Check sheet for the drawn part. Datum: minimum x, y, z corner. Units: mm. Coordinates: 2 decimals unless noted, no trailing zeros. Write each loop counter-clockwise with the first axis right and the second up, starting at its lowest first coordinate (ties: lowest second). Pieces come first, ordered by that corner, then holes. Notation, with made-up numbers: (83, 47) -> (93, 47) arc R20 cw to (93, 71) -> close; hole circle Ø3 at (25.25, 35.5). An arc over 180 degrees is marked (long way). Answer in a Markdown table with one row per item. Add a question column.
1. Scan lines: L1, parallel to X at y = 7, z = 1.75; L2, parallel to Y at x = 8.5, z = 0.6. Record each from-to range of solid material in increasing order. Write a range as from..to.
2. Cross-section at B-B on y = 1. Record the cut outline in (x, z).
3. Cross-section at A-A on y = 5. Record the cut outline in (x, z), and give its area (3 significant figures).
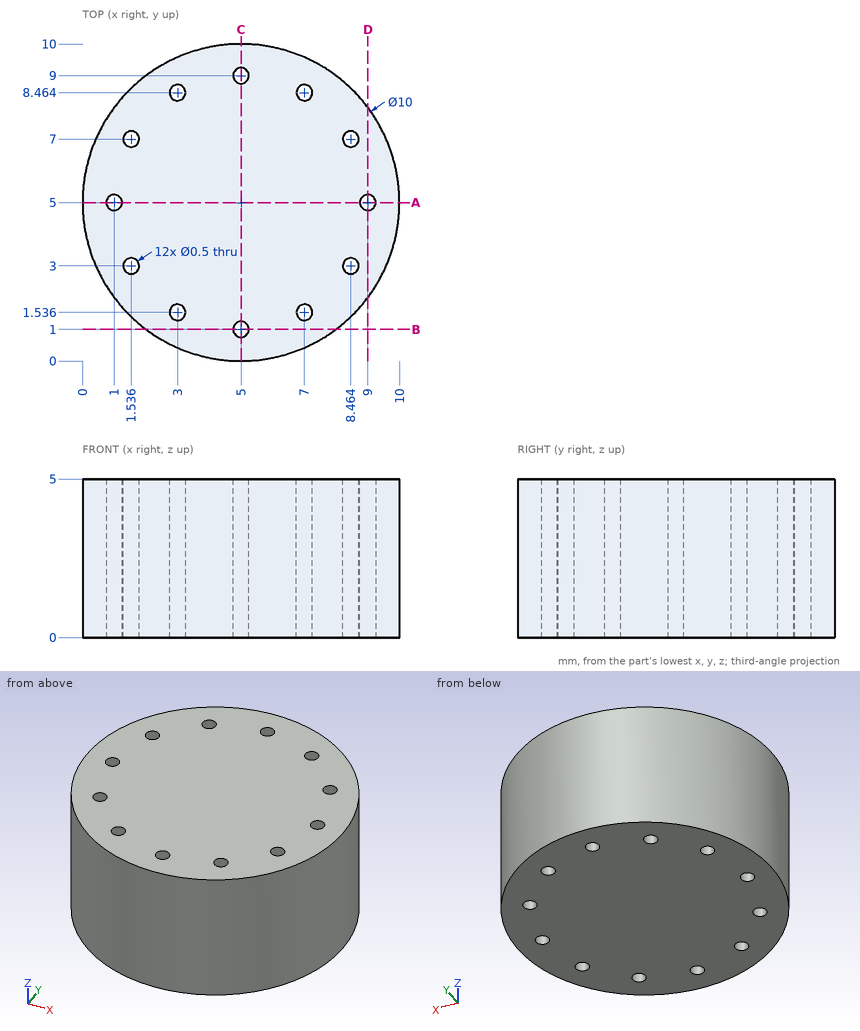
Results found:
| question | item | result |
|---|---|---|
| 1 | L1 | x = 0.42..1.29, 1.79..8.21, 8.71..9.58 |
| 1 | L2 | y = 1.43..2.75, 3.25..6.75, 7.25..8.57 |
| 2 | outline | (2, 0) -> (4.75, 0) -> (4.75, 5) -> (2, 5) -> close; (5.25, 0) -> (8, 0) -> (8, 5) -> (5.25, 5) -> close |
| 3 | outline | (0, 0) -> (0.75, 0) -> (0.75, 5) -> (0, 5) -> close; (1.25, 0) -> (8.75, 0) -> (8.75, 5) -> (1.25, 5) -> close; (9.25, 0) -> (10, 0) -> (10, 5) -> (9.25, 5) -> close |
| 3 | area | 45.0 mm^2 |
